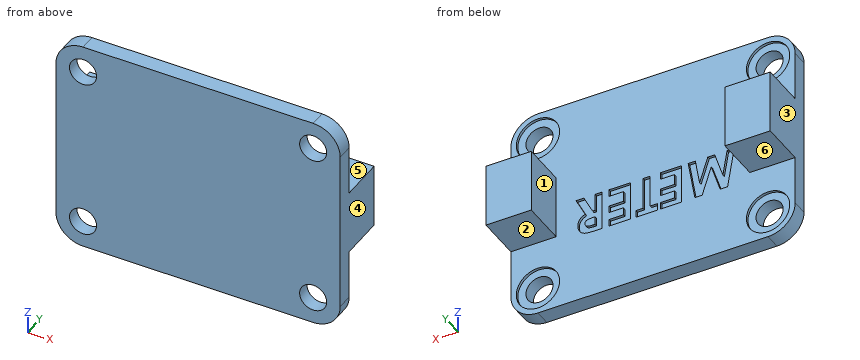
```python
from build123d import *

# Parameters (mm, degrees)
SKETCH1_W           = 26.67
SKETCH1_H           = 20.32
BOSS_EXTRUDE1_DEPTH = 1.5
SKETCH2_R           = 1.27
CUT_EXTRUDE1_DEPTH  = 17.831453443
FILLET1_R           = 2.54
CUT_EXTRUDE2_DEPTH  = 0.254
SKETCH4_R           = 2.032
SKETCH4_R_2         = 1.27
CUT_EXTRUDE3_DEPTH  = 0.254
SKETCH5_W           = 4.25
SKETCH5_H           = 6
BOSS_EXTRUDE3_DEPTH = 4.2


with BuildPart() as part:
    # Sketch1 → Boss-Extrude1 (new body)
    with BuildSketch(Plane(origin=(0, 0, 0), x_dir=(1, 0, 0), z_dir=(0, 1, 0))):
        Rectangle(SKETCH1_W, SKETCH1_H)
    extrude(amount=BOSS_EXTRUDE1_DEPTH)

    # Sketch2 → Cut-Extrude1 (cut, through all)
    with BuildSketch(Plane(origin=(0, 1.5, 0), x_dir=(1, 0, 0), z_dir=(0, 1, 0))):
        with Locations(Location((10.795, 7.62, 0), (0, 0, 270))):
            Circle(SKETCH2_R)
        with Locations(Location((-10.795, 7.62, 0), (0, 0, 270))):
            Circle(SKETCH2_R)
        with Locations(Location((-10.795, -7.62, 0), (0, 0, 270))):
            Circle(SKETCH2_R)
        with Locations(Location((10.795, -7.62, 0), (0, 0, 270))):
            Circle(SKETCH2_R)
    extrude(amount=-CUT_EXTRUDE1_DEPTH, mode=Mode.SUBTRACT)

    # Fillet1
    fillet1_edges = [part.edges().sort_by_distance(p)[0] for p in [
        (13.335, 0.75, 10.16),
        (-13.335, 0.75, 10.16),
        (-13.335, 0.75, -10.16),
        (13.335, 0.75, -10.16),
    ]]
    fillet(fillet1_edges, radius=FILLET1_R)

    # Sketch3 → Cut-Extrude2 (cut)
    # profile 1 of 5: a face of its own
    with BuildSketch(Plane(origin=(0, 1.5, 0), x_dir=(1, 0, 0), z_dir=(0, 1, 0))):
        Polygon((-6.996511919, 3.704166667), (-6.306432792, 3.704166667), (-5.461271368, 1.120451055), (-4.610173778, 3.704166667), (-3.926772837, 3.704166667), (-3.300507479, 0), (-3.973520132, 0), (-4.369017094, 2.339590845), (-5.139234442, 0), (-5.787760417, 0), (-6.553525641, 2.339590845), (-6.948280582, 0), (-7.622035256, 0), align=None)
    # profile 2 of 5: a face of its own
    with BuildSketch(Plane(origin=(0, 1.5, 0), x_dir=(1, 0, 0), z_dir=(0, 1, 0))):
        Polygon((-2.683146368, 3.704166667), (-0.688595085, 3.704166667), (-0.688595085, 3.039316239), (-2.01829594, 3.039316239), (-2.01829594, 2.326976496), (-0.688595085, 2.326976496), (-0.688595085, 1.662126068), (-2.01829594, 1.662126068), (-2.01829594, 0.664850427), (-0.688595085, 0.664850427), (-0.688595085, 0), (-2.683146368, 0), align=None)
    # profile 3 of 5: a face of its own
    with BuildSketch(Plane(origin=(0, 1.5, 0), x_dir=(1, 0, 0), z_dir=(0, 1, 0))):
        Polygon((-0.403659188, 3.704166667), (1.590892094, 3.704166667), (1.590892094, 3.039316239), (0.926041667, 3.039316239), (0.926041667, 0), (0.261191239, 0), (0.261191239, 3.039316239), (-0.403659188, 3.039316239), align=None)
    # profile 4 of 5: a face of its own
    with BuildSketch(Plane(origin=(0, 1.5, 0), x_dir=(1, 0, 0), z_dir=(0, 1, 0))):
        Polygon((2.113274573, 3.704166667), (4.107825855, 3.704166667), (4.107825855, 3.039316239), (2.778125, 3.039316239), (2.778125, 2.326976496), (4.107825855, 2.326976496), (4.107825855, 1.662126068), (2.778125, 1.662126068), (2.778125, 0.664850427), (4.107825855, 0.664850427), (4.107825855, 0), (2.113274573, 0), align=None)
    # profile 5 of 5: a face of its own
    with BuildSketch(Plane(origin=(0, 1.5, 0), x_dir=(1, 0, 0), z_dir=(0, 1, 0))):
        with BuildLine():
            Line((4.772676282, 3.704166667), (5.547345753, 3.704166667))
            add(Edge.make_bspline(
                [(5.547345753, 3.704166667), (5.598551169, 3.703984917), (5.697033609, 3.703635361), (5.839039907, 3.698120291), (5.969492221, 3.690445618), (6.088583697, 3.678733864), (6.196263387, 3.663205494), (6.292639209, 3.644900116), (6.377708347, 3.624037212), (6.452188242, 3.598040388), (6.519402665, 3.568716365), (6.582055851, 3.535022525), (6.641530024, 3.497334059), (6.697427662, 3.454659282), (6.75023453, 3.407765903), (6.800050251, 3.356606718), (6.846170881, 3.30074792), (6.888310842, 3.240542464), (6.926718023, 3.177207705), (6.960661917, 3.110656684), (6.988265147, 3.040843118), (7.01265556, 2.968775966), (7.030223185, 2.893425013), (7.04244121, 2.815523813), (7.051386771, 2.734798146), (7.051901098, 2.679956711), (7.052163462, 2.651981504)],
                knots=[0, 0, 0, 0, 1.749336639, 3.364467119, 4.854658419, 6.213483162, 7.451590619, 8.570285859, 9.5643256, 10.440900261, 11.26203566, 12.067320669, 12.869050712, 13.665104639, 14.467235401, 15.27997916, 16.102287765, 16.939272006, 17.78853747, 18.631303466, 19.488103222, 20.351255419, 21.228522269, 22.127379805, 23.044756219, 24, 24, 24, 24], degree=3))
            add(Edge.make_bspline(
                [(7.052163462, 2.651981504), (7.051481935, 2.622781813), (7.050145585, 2.565526543), (7.04294728, 2.481423219), (7.029791039, 2.400959043), (7.009863997, 2.324369601), (6.986960451, 2.250701651), (6.95650461, 2.18131441), (6.922132184, 2.115198744), (6.881309057, 2.053289882), (6.83650767, 1.994212705), (6.784404599, 1.940230679), (6.728375323, 1.888442475), (6.665270232, 1.842091929), (6.597871057, 1.798044986), (6.524838649, 1.758126726), (6.44664964, 1.721333695), (6.391678895, 1.700815359), (6.363568376, 1.69032285)],
                knots=[0, 0, 0, 0, 1.099860209, 2.156625411, 3.176576793, 4.16617041, 5.135385252, 6.078461593, 7.016046972, 7.938469504, 8.868247731, 9.803980173, 10.76021508, 11.73834243, 12.748633912, 13.790971185, 14.870363756, 16, 16, 16, 16], degree=3))
            Line((6.363568376, 1.69032285), (7.218376068, 0))
            Line((7.218376068, 0), (6.479323584, 0))
            Line((6.479323584, 0), (5.663100962, 1.614636752))
            Line((5.663100962, 1.614636752), (5.437526709, 1.614636752))
            Line((5.437526709, 1.614636752), (5.437526709, 0))
            Line((5.437526709, 0), (4.772676282, 0))
            Line((4.772676282, 0), (4.772676282, 3.704166667))
        make_face()
        with BuildLine():
            Line((5.437526709, 2.279487179), (5.696491887, 2.279487179))
            add(Edge.make_bspline(
                [(5.696491887, 2.279487179), (5.728152533, 2.279843763), (5.788775866, 2.280526544), (5.875960182, 2.283693564), (5.955144333, 2.291324517), (6.026668362, 2.300965941), (6.090892173, 2.312098358), (6.147242912, 2.328051787), (6.196588856, 2.34514629), (6.238345256, 2.366390323), (6.274020965, 2.390549396), (6.304824656, 2.417994704), (6.330303725, 2.449759153), (6.351274298, 2.484979522), (6.367587124, 2.523967328), (6.379494238, 2.566294572), (6.386148553, 2.612443416), (6.386914155, 2.644292402), (6.387313034, 2.660885751)],
                knots=[0, 0, 0, 0, 1.688639943, 3.233382647, 4.650958383, 5.928841754, 7.082724185, 8.122798841, 9.049171256, 9.863274652, 10.613301712, 11.341792392, 12.054588806, 12.776240173, 13.521029143, 14.301969904, 15.115324896, 16, 16, 16, 16], degree=3))
            add(Edge.make_bspline(
                [(6.387313034, 2.660885751), (6.386558917, 2.680516893), (6.385077593, 2.719078635), (6.370378255, 2.774594022), (6.346980086, 2.825977311), (6.314907604, 2.872996339), (6.274516483, 2.914216465), (6.228164484, 2.950552334), (6.174851221, 2.979284021), (6.125487151, 2.998235136), (6.080577385, 3.009573783), (6.040047739, 3.018023243), (5.993114165, 3.024011617), (5.93974123, 3.030363355), (5.880064984, 3.034482135), (5.813760155, 3.037488023), (5.741017172, 3.03871788), (5.690308404, 3.039111043), (5.663842982, 3.039316239)],
                knots=[0, 0, 0, 0, 1.020303359, 2.004196876, 2.966617323, 3.9489082, 4.950758222, 5.960522915, 7.003732012, 8.091992268, 8.70421221, 9.413913587, 10.24622431, 11.166358409, 12.212345909, 13.359657661, 14.621978493, 16, 16, 16, 16], degree=3))
            Line((5.663842982, 3.039316239), (5.437526709, 3.039316239))
            Line((5.437526709, 3.039316239), (5.437526709, 2.279487179))
        make_face(mode=Mode.SUBTRACT)
    extrude(amount=-CUT_EXTRUDE2_DEPTH, mode=Mode.SUBTRACT)

    # Sketch4 → Cut-Extrude3 (cut)
    # profile 1 of 4: a face of its own
    with BuildSketch(Plane(origin=(0, 1.5, 0), x_dir=(1, 0, 0), z_dir=(0, 1, 0))):
        with Locations(Location((-10.795, 7.62, 0), (0, 0, 270))):
            Circle(SKETCH4_R)
        with Locations(Location((-10.795, 7.62, 0), (0, 0, 270))):
            Circle(SKETCH4_R_2, mode=Mode.SUBTRACT)
    # profile 2 of 4: a face of its own
    with BuildSketch(Plane(origin=(0, 1.5, 0), x_dir=(1, 0, 0), z_dir=(0, 1, 0))):
        with Locations(Location((10.795, 7.62, 0), (0, 0, 270))):
            Circle(SKETCH4_R)
        with Locations(Location((10.795, 7.62, 0), (0, 0, 270))):
            Circle(SKETCH4_R_2, mode=Mode.SUBTRACT)
    # profile 3 of 4: a face of its own
    with BuildSketch(Plane(origin=(0, 1.5, 0), x_dir=(1, 0, 0), z_dir=(0, 1, 0))):
        with Locations(Location((10.795, -7.62, 0), (0, 0, 270))):
            Circle(SKETCH4_R)
        with Locations(Location((10.795, -7.62, 0), (0, 0, 270))):
            Circle(SKETCH4_R_2, mode=Mode.SUBTRACT)
    # profile 4 of 4: a face of its own
    with BuildSketch(Plane(origin=(0, 1.5, 0), x_dir=(1, 0, 0), z_dir=(0, 1, 0))):
        with Locations(Location((-10.795, -7.62, 0), (0, 0, 270))):
            Circle(SKETCH4_R)
        with Locations(Location((-10.795, -7.62, 0), (0, 0, 270))):
            Circle(SKETCH4_R_2, mode=Mode.SUBTRACT)
    extrude(amount=-CUT_EXTRUDE3_DEPTH, mode=Mode.SUBTRACT)

    # Sketch5 → Boss-Extrude3 (add)
    with BuildSketch(Plane(origin=(0, 1.5, 0), x_dir=(1, 0, 0), z_dir=(0, 1, 0))):
        with Locations((-11.21, 0)):
            Rectangle(SKETCH5_W, SKETCH5_H)
        with Locations((11.21, 0)):
            Rectangle(SKETCH5_W, SKETCH5_H)
    extrude(amount=BOSS_EXTRUDE3_DEPTH)


solid = part.part
```
Model file for the job. Use its own axes, mm. Face numbers are marked on the shaded views. A direction names the side the tool comes from. Give positions to 0.01 mm unless a question says otherwise; leave off trailing zeros. Write each loop counter-clockwise with the first axis right and the second up, starting at its lowest first coordinate (ties: lowest second). Pieces come first, ordered by that corner, then holes. Notation, with made-up numbers: M -2.5,51.5 L 51.5,51.5 A12 ccw 51.5,68.5 Z; hole C 87.25,50.5 d11. An arc over 180 degrees is marked long. Use a Markdown table: item, result.
1) Tool access for the marked faces 4, 5 and 6: list every direction of +Z, -Z, +X, -X, +Y, -Y with a clear straight run to the whole face (end or side of a thin tool).
Responses:
| item | result |
|---|---|
| face 4 | +Z, -Z, +X, +Y, -Y |
| face 5 | +Z, +X, -X, +Y |
| face 6 | -Z, +X, -X, +Y |
2) Cut at C-C (z = 0.5). List the corners of the cut face in (x, y) (3 decimals).
Responses:
| item | result |
|---|---|
| outline | M -13.335,0 L 13.335,0 L 13.335,5.7 L 9.085,5.7 L 9.085,1.5 L -9.085,1.5 L -9.085,5.7 L -13.335,5.7 Z |
3) Cut at B-B (z = -6.75). List the corners of the cut face in (x, y) (3 decimals), and give its area (3 significant figures).
Responses:
| item | result |
|---|---|
| outline | M -13.335,0 L -11.72,0 L -11.72,1.246 L -12.631,1.246 L -12.631,1.5 L -13.335,1.5 Z; M -9.87,0 L 9.87,0 L 9.87,1.246 L 8.959,1.246 L 8.959,1.5 L -8.959,1.5 L -8.959,1.246 L -9.87,1.246 Z; M 11.72,0 L 13.335,0 L 13.335,1.5 L 12.631,1.5 L 12.631,1.246 L 11.72,1.246 Z |
| area | 33.5 mm2 |
4) Drill centre lines: line 1 (X direction, y = 1.4, z = -7.62) (3 decimals); line 2 (X direction, y = 0.75, z = -7.62) (3 decimals); line 3 (X direction, y = 1.8, z = -0.5) (3 decimals). Where is each one in solid material? Low to high. Write a range as from..to.
Responses:
| item | result |
|---|---|
| line 1 | x = -13.335..-12.827, -8.763..8.763, 12.827..13.335 |
| line 2 | x = -13.335..-12.065, -9.525..9.525, 12.065..13.335 |
| line 3 | x = -13.335..-9.085, 9.085..13.335 |
5) Pin check, flat tips, straight feed: pin 1 (6 mm diameter, centred on x = -8.5, z = -4, fed in from +Y); pin 2 (1 mm diameter, centred on x = -4, y = 3.5, fed in from -Z); pin 3 (1.6 mm diameter, centred on x = 0.5, z = -1, fed in from +Y); pin 4 (2 mm diameter, centred on x = 11.5, z = -7, fed in from +Y). Stop position of each tip, or through.
Responses:
| item | result |
|---|---|
| pin 1 | stops at y = 5.7 |
| pin 2 | passes through |
| pin 3 | stops at y = 1.5 |
| pin 4 | stops at y = 1.25 |
6) Pull direction X, two halves, no side cores. Call the marked faces 1, 2 and 3: +X half, -X half, draft (parallel to the pull), parting line (faces both ways), or undercut.
Responses:
| item | result |
|---|---|
| face 1 | undercut |
| face 2 | draft |
| face 3 | -X half |
7) Cut at D-D (x = -10). List the corners of the cut face in (y, z).
Responses:
| item | result |
|---|---|
| outline | M 0,-10.16 L 1.5,-10.16 L 1.5,-9.49 L 1.25,-9.49 L 1.25,-8.61 L 0,-8.61 Z; M 0,-6.63 L 1.25,-6.63 L 1.25,-5.75 L 1.5,-5.75 L 1.5,-3 L 5.7,-3 L 5.7,3 L 1.5,3 L 1.5,5.75 L 1.25,5.75 L 1.25,6.63 L 0,6.63 Z; M 0,8.61 L 1.25,8.61 L 1.25,9.49 L 1.5,9.49 L 1.5,10.16 L 0,10.16 Z |
8) Cut at A-A (y = 3.35). List the corners of the cut face in (x, z) (3 decimals).
Responses:
| item | result |
|---|---|
| outline | M -13.335,-3 L -9.085,-3 L -9.085,3 L -13.335,3 Z; M 9.085,-3 L 13.335,-3 L 13.335,3 L 9.085,3 Z |
